Work out the finished part from the listing and answer in its coordinate system (mm). A direction names the side the tool comes from. Give positions to 0.01 mm unless a question says otherwise; leave off trailing zeros. Use one line per item in the form item = value. Start each with the question number.
from build123d import *

# Parameters (mm, degrees)
F0_W          = 24
F0_H          = 116
F1_DEPTH      = 44
F2_T          = -3
F3_W          = 8.5
F3_H          = 16.5
F3_W_2        = 10.6
F3_H_2        = 12.5
F4_DEPTH      = 25
F5_W          = 6
F5_H          = 15.5
F6_DEPTH      = 25
F7_SIZE2      = 2.25
F7_SIZE       = 1.5
F9_DEPTH      = 7
F10_R         = 2.4
F11_DEPTH     = 1.6
F12_R         = 2
F13_T1_DEPTH  = 47
F13_S5_W      = 2
F13_S5_H      = 2
F13_T6_DEPTH  = 2
F13_S11_W     = 2
F13_S11_H     = 2
F13_T12_DEPTH = 2
F13_S17_W     = 2
F13_S17_H     = 2
F13_T18_DEPTH = 2
F13_S23_W     = 2
F13_S23_H     = 2
F13_T24_DEPTH = 2


# Not quite as in the source:
# - a fillet or chamfer that OpenCascade refuses, or shapes differently, is made with other operations: its cross-section is extruded or revolved along the edge and cut away or added


with BuildPart() as f1:
    # F0 (on Top) → F1 (new body)
    with BuildSketch(Plane.XY):
        Rectangle(F0_W, F0_H)
    extrude(amount=F1_DEPTH)

    # F2
    f2_openings = [f1.faces().sort_by_distance(p)[0] for p in [
        (0, 0, 44),
    ]]
    offset(amount=F2_T, openings=f2_openings)

    # F3 (on face) → F4 (cut)
    with BuildSketch(Plane(origin=(0, 0, 0), x_dir=(1, 0, 0), z_dir=(0, 0, -1))):
        with Locations((-4.75, 9.75)):
            Rectangle(F3_W, F3_H)
        with Locations((-3.7, -11.75)):
            Rectangle(F3_W_2, F3_H_2)
    extrude(amount=-F4_DEPTH, mode=Mode.SUBTRACT)

    # F5 (on face) → F6 (cut)
    with BuildSketch(Plane(origin=(0, 58, 0), x_dir=(-1, 0, 0), z_dir=(0, 1, 0))):
        with Locations((4, 31.25)):
            Rectangle(F5_W, F5_H)
    extrude(amount=-F6_DEPTH, mode=Mode.SUBTRACT)

    # F7
    f7_edges = [f1.edges().sort_by_distance(p)[0] for p in [
        (-1, 56.5, 23.5),
        (-1, 56.5, 39),
    ]]
    chamfer(f7_edges, length=F7_SIZE, length2=F7_SIZE2)

    # F8 (on face) → F9 (join)
    with BuildSketch(Plane.XY.offset(3)):
        Polygon((4.6, 21), (-9, 21), (-9, 18), (1.6, 18), (1.6, 5.5), (-9, 5.5), (-9, 2.5), (4.6, 2.5), align=None)
        Polygon((-9, -18), (-9, -21), (2.5, -21), (2.5, 1.5), (-9, 1.5), (-9, -1.5), (-0.5, -1.5), (-0.5, -18), align=None)
    extrude(amount=F9_DEPTH)

    # F10 (on face) → F11 (join)
    with BuildSketch(Plane(origin=(-12, 0, 0), x_dir=(0, -1, 0), z_dir=(-1, 0, 0))):
        with Locations((-52, 6)):
            Circle(F10_R)
        with Locations((-52, 14)):
            Circle(F10_R)
        with Locations((-52, 22)):
            Circle(F10_R)
        with Locations((-52, 30)):
            Circle(F10_R)
        with Locations((-52, 38)):
            Circle(F10_R)
        with Locations((-44, 6)):
            Circle(F10_R)
        with Locations((-44, 14)):
            Circle(F10_R)
        with Locations((-44, 22)):
            Circle(F10_R)
        with Locations((-44, 30)):
            Circle(F10_R)
        with Locations((-44, 38)):
            Circle(F10_R)
        with Locations((-36, 6)):
            Circle(F10_R)
        with Locations((-36, 14)):
            Circle(F10_R)
        with Locations((-36, 22)):
            Circle(F10_R)
        with Locations((-36, 30)):
            Circle(F10_R)
        with Locations((-36, 38)):
            Circle(F10_R)
        with Locations((-28, 6)):
            Circle(F10_R)
        with Locations((-28, 14)):
            Circle(F10_R)
        with Locations((-28, 22)):
            Circle(F10_R)
        with Locations((-28, 30)):
            Circle(F10_R)
        with Locations((-28, 38)):
            Circle(F10_R)
        with Locations((-20, 6)):
            Circle(F10_R)
        with Locations((-20, 14)):
            Circle(F10_R)
        with Locations((-20, 22)):
            Circle(F10_R)
        with Locations((-20, 30)):
            Circle(F10_R)
        with Locations((-20, 38)):
            Circle(F10_R)
        with Locations((-12, 6)):
            Circle(F10_R)
        with Locations((-12, 14)):
            Circle(F10_R)
        with Locations((-12, 22)):
            Circle(F10_R)
        with Locations((-12, 30)):
            Circle(F10_R)
        with Locations((-12, 38)):
            Circle(F10_R)
        with Locations((-4, 6)):
            Circle(F10_R)
        with Locations((-4, 14)):
            Circle(F10_R)
        with Locations((-4, 22)):
            Circle(F10_R)
        with Locations((-4, 30)):
            Circle(F10_R)
        with Locations((-4, 38)):
            Circle(F10_R)
        with Locations((4, 6)):
            Circle(F10_R)
        with Locations((4, 14)):
            Circle(F10_R)
        with Locations((4, 22)):
            Circle(F10_R)
        with Locations((4, 30)):
            Circle(F10_R)
        with Locations((4, 38)):
            Circle(F10_R)
        with Locations((12, 6)):
            Circle(F10_R)
        with Locations((12, 14)):
            Circle(F10_R)
        with Locations((12, 22)):
            Circle(F10_R)
        with Locations((12, 30)):
            Circle(F10_R)
        with Locations((12, 38)):
            Circle(F10_R)
        with Locations((20, 6)):
            Circle(F10_R)
        with Locations((20, 14)):
            Circle(F10_R)
        with Locations((20, 22)):
            Circle(F10_R)
        with Locations((20, 30)):
            Circle(F10_R)
        with Locations((20, 38)):
            Circle(F10_R)
        with Locations((28, 6)):
            Circle(F10_R)
        with Locations((28, 14)):
            Circle(F10_R)
        with Locations((28, 22)):
            Circle(F10_R)
        with Locations((28, 30)):
            Circle(F10_R)
        with Locations((28, 38)):
            Circle(F10_R)
        with Locations((36, 6)):
            Circle(F10_R)
        with Locations((36, 14)):
            Circle(F10_R)
        with Locations((36, 22)):
            Circle(F10_R)
        with Locations((36, 30)):
            Circle(F10_R)
        with Locations((36, 38)):
            Circle(F10_R)
        with Locations((44, 6)):
            Circle(F10_R)
        with Locations((44, 14)):
            Circle(F10_R)
        with Locations((44, 22)):
            Circle(F10_R)
        with Locations((44, 30)):
            Circle(F10_R)
        with Locations((44, 38)):
            Circle(F10_R)
        with Locations((52, 6)):
            Circle(F10_R)
        with Locations((52, 14)):
            Circle(F10_R)
        with Locations((52, 22)):
            Circle(F10_R)
        with Locations((52, 30)):
            Circle(F10_R)
        with Locations((52, 38)):
            Circle(F10_R)
    extrude(amount=F11_DEPTH)

    # F12
    f12_edges = [f1.edges().sort_by_distance(p)[0] for p in [
        (12, 0, 0),
        (0, -58, 0),
        (-12, 0, 0),
        (0, 58, 0),
    ]]
    fillet(f12_edges, radius=F12_R)

    # F13: fillet of radius 2 on 4 edges, made by hand

    # F13_s2 → F13_t1 (cut)
    with BuildSketch(Plane.XY.offset(2)):
        with BuildLine():
            ThreePointArc((-12, -56), (-11.4142135624, -57.4142135624), (-10, -58))
            Line((-10, -58), (-12, -58))
            Line((-12, -58), (-12, -56))
        make_face()
        with BuildLine():
            ThreePointArc((12, -56), (11.4142135624, -57.4142135624), (10, -58))
            Line((10, -58), (12, -58))
            Line((12, -58), (12, -56))
        make_face()
        with BuildLine():
            ThreePointArc((10, 58), (11.4142135624, 57.4142135624), (12, 56))
            Line((12, 56), (12, 58))
            Line((12, 58), (10, 58))
        make_face()
        with BuildLine():
            ThreePointArc((-10, 58), (-11.4142135624, 57.4142135624), (-12, 56))
            Line((-12, 56), (-12, 58))
            Line((-12, 58), (-10, 58))
        make_face()
    extrude(amount=F13_T1_DEPTH, mode=Mode.SUBTRACT)


with BuildPart() as f13_tool4:
    # F13_s5 → F13_t6 (new body)
    with BuildSketch(Plane.XZ.offset(-56)):
        with Locations((-11, 1)):
            Rectangle(F13_S5_W, F13_S5_H)
    extrude(amount=-F13_T6_DEPTH)

    # F13_s7 → F13_t8 (revolve, cut)
    with BuildSketch(Plane(origin=(-10, 56, 2), x_dir=(0.7071067812, 0, 0.7071067812), z_dir=(-0.7071067812, 0, 0.7071067812))):
        with BuildLine():
            ThreePointArc((0, -2), (2, 0), (0, 2))
            Line((0, 2), (0, -2))
        make_face()
    revolve(axis=Axis((-10, 56, 2), (0, 1, 0)), mode=Mode.SUBTRACT)


with BuildPart() as f1_1:
    add(f1.part)

    # F13_t3: cut F13_tool4
    add(f13_tool4.part, mode=Mode.SUBTRACT)


with BuildPart() as f13_tool10:
    # F13_s11 → F13_t12 (new body)
    with BuildSketch(Plane.XZ.offset(-56)):
        with Locations((11, 1)):
            Rectangle(F13_S11_W, F13_S11_H)
    extrude(amount=-F13_T12_DEPTH)

    # F13_s13 → F13_t14 (revolve, cut)
    with BuildSketch(Plane(origin=(10, 56, 2), x_dir=(-0.7071067812, 0, 0.7071067812), z_dir=(-0.7071067812, 0, -0.7071067812))):
        with BuildLine():
            ThreePointArc((0, -2), (2, 0), (0, 2))
            Line((0, 2), (0, -2))
        make_face()
    revolve(axis=Axis((10, 56, 2), (0, 1, 0)), mode=Mode.SUBTRACT)


with BuildPart() as f1_2:
    add(f1_1.part)

    # F13_t9: cut F13_tool10
    add(f13_tool10.part, mode=Mode.SUBTRACT)


with BuildPart() as f13_tool16:
    # F13_s17 → F13_t18 (new body)
    with BuildSketch(Plane.YZ.offset(10)):
        with Locations((-57, 1)):
            Rectangle(F13_S17_W, F13_S17_H)
    extrude(amount=F13_T18_DEPTH)

    # F13_s19 → F13_t20 (revolve, cut)
    with BuildSketch(Plane(origin=(10, -56, 2), x_dir=(0, 0.7071067812, 0.7071067812), z_dir=(0, 0.7071067812, -0.7071067812))):
        with BuildLine():
            ThreePointArc((0, -2), (2, 0), (0, 2))
            Line((0, 2), (0, -2))
        make_face()
    revolve(axis=Axis((10, -56, 2), (1, 0, 0)), mode=Mode.SUBTRACT)


with BuildPart() as f1_3:
    add(f1_2.part)

    # F13_t15: cut F13_tool16
    add(f13_tool16.part, mode=Mode.SUBTRACT)


with BuildPart() as f13_tool22:
    # F13_s23 → F13_t24 (new body)
    with BuildSketch(Plane.YZ.offset(-10)):
        with Locations((-57, 1)):
            Rectangle(F13_S23_W, F13_S23_H)
    extrude(amount=-F13_T24_DEPTH)

    # F13_s25 → F13_t26 (revolve, cut)
    with BuildSketch(Plane(origin=(-10, -56, 2), x_dir=(0, 0.7071067812, 0.7071067812), z_dir=(0, -0.7071067812, 0.7071067812))):
        with BuildLine():
            ThreePointArc((0, -2), (2, 0), (0, 2))
            Line((0, 2), (0, -2))
        make_face()
    revolve(axis=Axis((-10, -56, 2), (-1, 0, 0)), mode=Mode.SUBTRACT)


with BuildPart() as f1_4:
    add(f1_3.part)

    # F13_t21: cut F13_tool22
    add(f13_tool22.part, mode=Mode.SUBTRACT)


solid = f1_4.part
1) A tool of negligible diameter and unlimited length cuts with its end or side. For faces 1 (the flat face through (9, -1, 23)), 2 (the cylindrical face through (-12.79, 18.89, 35.87)), 3 (the flat face through (-1.74, 56.52, 24.64)), from which of +Z, -Z, +X, -X, +Y, -Y can it reach the whole face along a straight path? Write none if from no direction.
2) Determine the mould class of faces 4 (the cylindrical face through (-12.789, 12.52, 35.657)), 5 (the cylindrical face through (-11.43, -57.4, 22.71)), 6 (the flat face through (2, 14, 10)) for opening direction Z: released by +Z, released by -Z, zero draft, split by the parting line, or undercut.
3) A cutting plane is placed at A-A (x = -5). State how many separate pieces and enclosed holes the cut face has, plus the area to 3 significant figures.
4) A flat-ended cylindrical pin translates along its axis: pin 1 Ø5.5 at (x, y) = (0, -6) entering from +Z. Find the tip coordinate at first contact, or state that the pin passes through.
5) Find the intervals of material crossed by probe 1 along Y at (x, z) = (-1.75, 6.5); probe 2 along Y at (x, z) = (0.25, 2); probe 3 along Y at (x, z) = (-7.5, 30), in increasing order.
Answer sheet:
q1.face_1 = +Z
q1.face_2 = -X
q1.face_3 = +Y
q2.face_4 = undercut
q2.face_5 = zero draft
q2.face_6 = released by +Z
q3.separate_pieces = 4
q3.enclosed_holes = 0
q3.area = 543 mm²
q4.pin_1 = 10
q5.probe_1 = -58 to -55, -21 to -18, -1.5 to 1.5, 2.5 to 5.5, 18 to 21, 55 to 58
q5.probe_2 = -58 to 5.5, 18 to 58
q5.probe_3 = -58 to -55, 55 to 58
